```python
from build123d import *

# Parameters (mm, degrees)
F0_W            = 210
F0_H            = 225
F1_DEPTH        = 25
F3_DEPTH        = 95
F4_R            = 37.5
F5_DEPTH        = 10
F5_DEPTH_BACK   = 127
F6_R            = 40
F7_DEPTH        = 10
F7_DEPTH_BACK   = 127
F8_W            = 60
F8_H            = 60
F9_DEPTH        = 10
F10_R           = 10
F12_DEPTH       = 20
F14_D           = 15
F14_CBORE_D     = 30
F14_CBORE_DEPTH = 10
F15_R           = 10
F16_R           = 19.5
F17_DEPTH       = 235.001
F18_R           = 19.5
F19_DEPTH       = 220.001
F20_SIZE        = 2
F21_R           = 10


with BuildPart() as f1:
    # F0 (on Top) → F1 (new body)
    with BuildSketch(Plane.XY):
        Rectangle(F0_W, F0_H)
    extrude(amount=F1_DEPTH)

    # F2 (on face) → F3 (join)
    with BuildSketch(Plane.XY.offset(25)):
        with BuildLine():
            Line((-71, -32.5), (-71, -112.5))
            Line((-71, -112.5), (-56, -112.5))
            Line((-56, -112.5), (-56, -46.481817))
            ThreePointArc((-56, -46.481817), (7.488853, -14.988853), (38.981817, 48.5))
            Line((38.981817, 48.5), (105, 48.5))
            Line((105, 48.5), (105, 63.5))
            Line((105, 63.5), (25, 63.5))
            ThreePointArc((25, 63.5), (-3.117749, -4.382251), (-71, -32.5))
        make_face()
    extrude(amount=F3_DEPTH)

    # F4 (on face) → F5 (join, two sides)
    with BuildSketch(Plane.XZ.offset(112.5)) as f5_sk:
        with Locations((-63.5, 120)):
            Circle(F4_R)
    extrude(amount=F5_DEPTH)
    extrude(f5_sk.sketch, amount=-F5_DEPTH_BACK)

    # F6 (on face) → F7 (join, two sides)
    with BuildSketch(Plane.YZ.offset(105)) as f7_sk:
        with Locations((56, 120)):
            Circle(F6_R)
    extrude(amount=F7_DEPTH)
    extrude(f7_sk.sketch, amount=-F7_DEPTH_BACK)

    # F8 (on face) → F9 (join)
    with BuildSketch(Plane.XY.offset(25)):
        with Locations((75, -82.5)):
            Rectangle(F8_W, F8_H)
    extrude(amount=F9_DEPTH)

    # F10
    f10_edges = [f1.edges().sort_by_distance(p)[0] for p in [
        (45, -52.5, 30),
    ]]
    fillet(f10_edges, radius=F10_R)

    # F11 (on face) → F12 (cut)
    with BuildSketch(Plane.XY.offset(25)):
        with BuildLine():
            ThreePointArc((43.262855, 43.5), (11.024387, -18.524387), (-51, -50.762855))
            Line((-51, -50.762855), (-51, -107.5))
            Line((-51, -107.5), (40, -107.5))
            Line((40, -107.5), (40, -62.5))
            ThreePointArc((40, -62.5), (44.393398, -51.893398), (55, -47.5))
            Line((55, -47.5), (100, -47.5))
            Line((100, -47.5), (100, 43.5))
            Line((100, 43.5), (43.262855, 43.5))
        make_face()
    extrude(amount=-F12_DEPTH, mode=Mode.SUBTRACT)

    # F14 (through all)
    with Locations(Plane.XY.offset(35)):
        with Locations((75, -82.5)):
            CounterBoreHole(F14_D / 2, F14_CBORE_D / 2, F14_CBORE_DEPTH)

    # F15
    f15_edges = [f1.edges().sort_by_distance(p)[0] for p in [
        (-51, -50.762855, 15),
        (43.262855, 43.5, 15),
        (100, 43.5, 15),
        (40, -107.5, 15),
        (100, -47.5, 15),
        (-51, -107.5, 15),
    ]]
    fillet(f15_edges, radius=F15_R)

    # F16 (on face) → F17 (cut, through all)
    with BuildSketch(Plane.XZ.offset(122.5)):
        with Locations((-63.5, 120)):
            Circle(F16_R)
    extrude(amount=-F17_DEPTH, mode=Mode.SUBTRACT)

    # F18 (on face) → F19 (cut, through all)
    with BuildSketch(Plane.YZ.offset(115)):
        with Locations((56, 120)):
            Circle(F18_R)
    extrude(amount=-F19_DEPTH, mode=Mode.SUBTRACT)

    # F20
    f20_edges = [f1.edges().sort_by_distance(p)[0] for p in [
        (-83, -122.5, 120),
        (115, 36.5, 120),
        (-22, 36.5, 120),
        (-83, 14.5, 120),
    ]]
    chamfer(f20_edges, length=F20_SIZE)

    # F21
    f21_edges = [f1.edges().sort_by_distance(p)[0] for p in [
        (-105, 112.5, 12.5),
        (-105, -112.5, 12.5),
        (105, 112.5, 12.5),
        (105, -112.5, 17.5),
    ]]
    fillet(f21_edges, radius=F21_R)


solid = f1.part
```
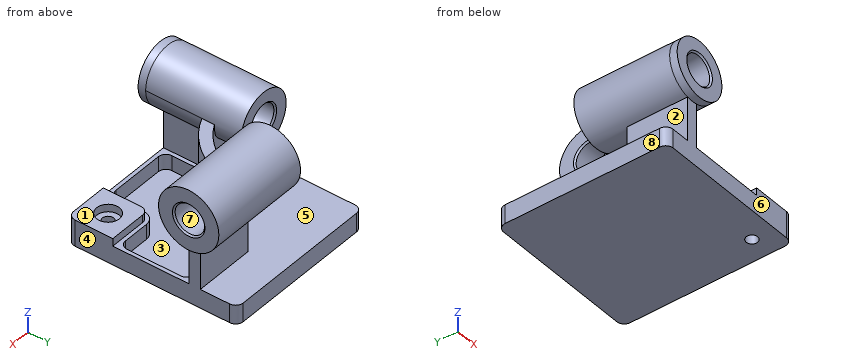
The listing builds one solid part. Answer for the finished solid, in the listing's coordinates (mm). Face numbers are marked on the shaded views. A direction names the side the tool comes from. Give positions to 0.01 mm unless a question says otherwise; leave off trailing zeros. Write each loop counter-clockwise with the first axis right and the second up, starting at its lowest first coordinate (ties: lowest second). Pieces come first, ordered by that corner, then holes. Notation, with made-up numbers: (48.5, -16.75) -> (52.5, -16.75) arc R27 cw to (52.5, 15.25) -> close; hole circle Ø8 at (87, -14). An arc over 180 degrees is marked (long way). Use one line per item in the form item = value.
1) Each of these flat-tipped pins is pushed along its axis until it touches: P1, Ø8, axis at x = 74, z = 136.5, coming from the -Y side; P2, Ø2, axis at x = -8.5, z = 130.5, coming from the -Y side; P3, Ø2, axis at x = -53.5, z = 54, coming from the -Y side. Where does it stop, or does it pass through?
Result:
P1 = 18
P2 = 17.14
P3 = -46.27
2) Section A-A on y = -82.5 is taken. Write down the section's boundary in (x, z).
Result:
outline = (-105, 0) -> (67.5, 0) -> (67.5, 25) -> (60, 25) -> (60, 35) -> (45, 35) -> (45, 25) -> (40, 25) -> (40, 5) -> (-51, 5) -> (-51, 25) -> (-56, 25) -> (-56, 83.26) arc R37.5 ccw (long way) to (-71, 83.26) -> (-71, 25) -> (-105, 25) -> close; (82.5, 0) -> (105, 0) -> (105, 35) -> (90, 35) -> (90, 25) -> (82.5, 25) -> close; hole circle Ø39 at (-63.5, 120)
3) Section D-D on z = 72 is taken. Write down the section's boundary in (x, y).
Result:
outline = (-71, -112.5) -> (-56, -112.5) -> (-56, -46.48) arc R111 ccw to (38.98, 48.5) -> (105, 48.5) -> (105, 63.5) -> (25, 63.5) arc R96 cw to (-71, -32.5) -> close
4) Section B-B on x = 75 is taken. Write down the section's boundary in (y, z).
Result:
outline = (-112.5, 0) -> (-90, 0) -> (-90, 25) -> (-97.5, 25) -> (-97.5, 35) -> (-112.5, 35) -> close; (-75, 0) -> (112.5, 0) -> (112.5, 25) -> (63.5, 25) -> (63.5, 80.71) arc R40 ccw (long way) to (48.5, 80.71) -> (48.5, 25) -> (43.5, 25) -> (43.5, 5) -> (-47.5, 5) -> (-47.5, 25) -> (-52.5, 25) -> (-52.5, 35) -> (-67.5, 35) -> (-67.5, 25) -> (-75, 25) -> close; hole circle Ø39 at (56, 120)
5) A tool of negligible diameter and unlimited length cuts with its end or side. For the marked faces 1, 2, 3, 4 and 5, from which of +Z, -Z, +X, -X, +Y, -Y can it reach the whole face along a straight path? Write none if from no direction.
Result:
face_1 = +Z, +X, -Y
face_2 = -X, +Y, -Y
face_3 = none
face_4 = -Z, +X, +Y, -Y
face_5 = -X, +Y
6) Straight lines are drawn through the part: probe 1 along X at (y, z) = (-82, 31); probe 2 along Y at (x, z) = (75, 28); probe 3 along Z at (x, y) = (23, 56). For each, find the intervals that lie inside material, in ascending order.
Result:
probe_1 = -71 to -56, 45 to 60.01, 89.99 to 105
probe_2 = -112.5 to -97.5, -67.5 to -52.5, 48.5 to 63.5
probe_3 = 0 to 25, 80 to 100.5, 139.5 to 160
7) Section C-C on x = -63.5 is taken. Write down the section's boundary in (y, z), plus the area to 3 significant figures.
Result:
outline = (-122.5, 82.5) -> (-112.5, 82.5) -> (-112.5, 0) -> (112.5, 0) -> (112.5, 25) -> (-32.21, 25) -> (-32.21, 82.5) -> (14.5, 82.5) -> (14.5, 98.5) -> (12.5, 100.5) -> (-120.5, 100.5) -> (-122.5, 98.5) -> close; (-122.5, 141.5) -> (-120.5, 139.5) -> (12.5, 139.5) -> (14.5, 141.5) -> (14.5, 157.5) -> (-122.5, 157.5) -> close
area = 15,200 mm²
8) For a pull along Y with two mould halves and no side action, classify the marked faces 6, 7 and 8 as +Y half, -Y half, draft (parallel to the pull), parting line (faces both ways), or undercut.
Result:
face_6 = -Y half
face_7 = undercut
face_8 = draft
